from build123d import *

# Parameters (mm, degrees)
F0_W     = 24
F0_H     = 24
F1_DEPTH = 25
F3_D     = 6


with BuildPart() as f1:
    # F0 (on Top) → F1 (new body)
    with BuildSketch(Plane.XY):
        with Locations((12, -12)):
            Rectangle(F0_W, F0_H)
    extrude(amount=F1_DEPTH)

    # F3 (through all)
    with Locations(Plane.XZ.offset(24)):
        with Locations((12, 20), (12, 10)):
            Hole(F3_D / 2)


solid = f1.part
Design review of the part built by this model. Coordinates are the model's own, in mm. Round coordinates to 2 decimals unless told otherwise and drop trailing zeros. Write each loop counter-clockwise with the first axis right and the second up, starting at its lowest first coordinate (ties: lowest second). Pieces come first, ordered by that corner, then holes. Notation, with made-up numbers: (-15, -31.75) - (-9, -31.75) arc R18 ccw to (-9, -21.75) - close; hole circle Ø4 at (19.25, 0). An arc over 180 degrees is marked (long way). Return JSON: item names as keys, results as strings. Group by question number.
Item 1: We need section A-A on z = 20. Write out the cut boundary in (x, y).
Item 2: Insertion check: P1, Ø3.5, axis at x = 12, z = 20, coming from the -Y side. The pin has a flat end and moves straight along its axis. Give the tip position at first contact, or say it passes through.
Item 3: The part is to be moulded in two halves that separate along X. For faces 1 (the face through (12, -12, 25)), 2 (the face through (0, -12, 12)), 3 (the face through (14.4, -11.8, 18.2)), 4 (the face through (14.4, -11.8, 8.2)), say which applies: pulls with the +X half, pulls with the -X half, needs draft (parallel to the pull), parting line crosses it, or undercut.
Item 4: We need section C-C on y = -15.5. Write out the cut boundary in (x, z), and give its area (3 significant figures).
Item 5: We need section B-B on x = 12. Write out the cut boundary in (y, z).
Item 6: For probe 1 along Z at (x, y) = (12, -14.75); probe 2 along Z at (x, y) = (9.5, -22); probe 3 along X at (y, z) = (-22, 19), list the stretches that pass through material, from the lowest coordinate up. Write a range as [from, to].
Model answer:
{
 "1": {"outline": "(0, -24) - (9, -24) - (9, 0) - (0, 0) - close; (15, -24) - (24, -24) - (24, 0) - (15, 0) - close"},
 "2": {"P1": "passes through"},
 "3": {"face 1": "needs draft", "face 2": "pulls with the -X half", "face 3": "undercut", "face 4": "undercut"},
 "4": {"outline": "(0, 0) - (24, 0) - (24, 25) - (0, 25) - close; hole circle Ø6 at (12, 10); hole circle Ø6 at (12, 20)", "area": "543 mm²"},
 "5": {"outline": "(-24, 0) - (0, 0) - (0, 7) - (-24, 7) - close; (-24, 13) - (0, 13) - (0, 17) - (-24, 17) - close; (-24, 23) - (0, 23) - (0, 25) - (-24, 25) - close"},
 "6": {"probe 1": "z = [0, 7], [13, 17], [23, 25]", "probe 2": "z = [0, 8.34], [11.66, 18.34], [21.66, 25]", "probe 3": "x = [0, 9.17], [14.83, 24]"}
}
